Build history of the part. All positions in model axes, mm. Face numbers are marked on the shaded views. Give positions to 0.01 mm unless a question says otherwise; leave off trailing zeros. Loops run counter-clockwise (first coordinate to the right, second up) from the corner with the lowest first, then second, coordinate; pieces in that order, holes last. Notation, with made-up numbers: (84, -18.75) -> (115, -18.75) arc R21 cw to (115, -4.75) -> close; hole circle Ø5 at (-27.5, 82.5). An arc over 180 degrees is marked (long way). Answer as a JSON object with one key per item and string values. Group by question number.
from build123d import *

# Parameters (mm, degrees)
SKETCH1_R           = 57.15
BOSS_EXTRUDE1_DEPTH = 190.5
BOSS_EXTRUDE1_TAPER = -1
SKETCH3_R           = 55.15
CUT_EXTRUDE1_DEPTH  = 190.5
CUT_EXTRUDE1_TAPER  = -1
SKETCH4_R           = 57.15
BOSS_EXTRUDE2_DEPTH = 2


with BuildPart() as part:
    # Sketch1 → Boss-Extrude1 (new body)
    with BuildSketch(Plane(origin=(0, 0, 0), x_dir=(1, 0, 0), z_dir=(0, 1, 0))):
        Circle(SKETCH1_R)
    extrude(amount=BOSS_EXTRUDE1_DEPTH, taper=BOSS_EXTRUDE1_TAPER)

    # Sketch3 → Cut-Extrude1 (cut)
    with BuildSketch(Plane.XZ):
        Circle(SKETCH3_R)
    extrude(amount=-CUT_EXTRUDE1_DEPTH, taper=CUT_EXTRUDE1_TAPER, mode=Mode.SUBTRACT)

    # Sketch4 → Boss-Extrude2 (add)
    with BuildSketch(Plane.XZ):
        Circle(SKETCH4_R)
    extrude(amount=BOSS_EXTRUDE2_DEPTH)


solid = part.part
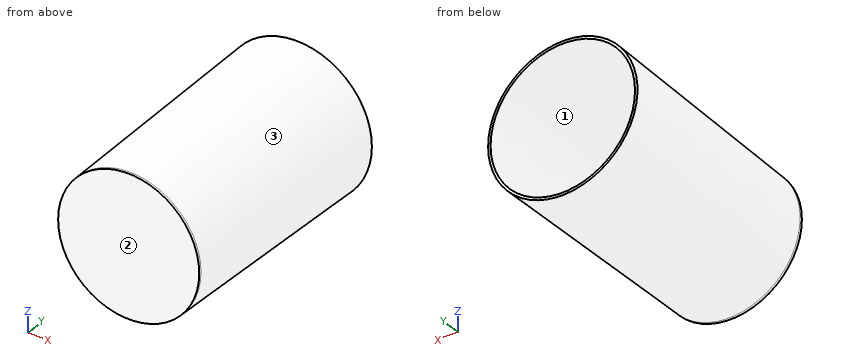
(1) Pin check, flat tips, straight feed: pin 1 (5 mm diameter, centred on x = -28, z = 28, fed in from +Y); pin 2 (8 mm diameter, centred on x = -30.5, y = 26, fed in from +Z); pin 3 (3 mm diameter, centred on x = 33, y = 75.5, fed in from +Z). Stop position of each tip, or through.
(2) Saw through at A-A on y = 61. List the corners of the cut face in (x, z).
(3) Saw through at B-B on y = 93. List the corners of the cut face in (x, z).
(4) Pull direction X, two halves, no side cores. Call the marked faces 1, 2 and 3: pulls with the +X half, pulls with the -X half, needs draft (parallel to the pull), parting line crosses it, or undercut.
(5) Probe line 1 along Y through (x, z) = (-14, -29.5); line 2 along X through (y, z) = (86, 16); line 3 along X through (y, z) = (142, -44.5). List the from-to ranges inside material, lowest first. Write a range as [from, to].
Calculated:
{
 "1": {"pin 1": "stops at y = 0", "pin 2": "stops at z = 51.15", "pin 3": "stops at z = 49.26"},
 "2": {"outline": "circle Ø116.43 at (0, 0); hole circle Ø112.43 at (0, 0)"},
 "3": {"outline": "circle Ø117.55 at (0, 0); hole circle Ø113.55 at (0, 0)"},
 "4": {"face 1": "undercut", "face 2": "needs draft", "face 3": "parting line crosses it"},
 "5": {"line 1": "y = [-2, 0]", "line 2": "x = [-56.43, -54.34], [54.34, 56.43]", "line 3": "x = [-39.69, -36.62], [36.62, 39.69]"}
}
